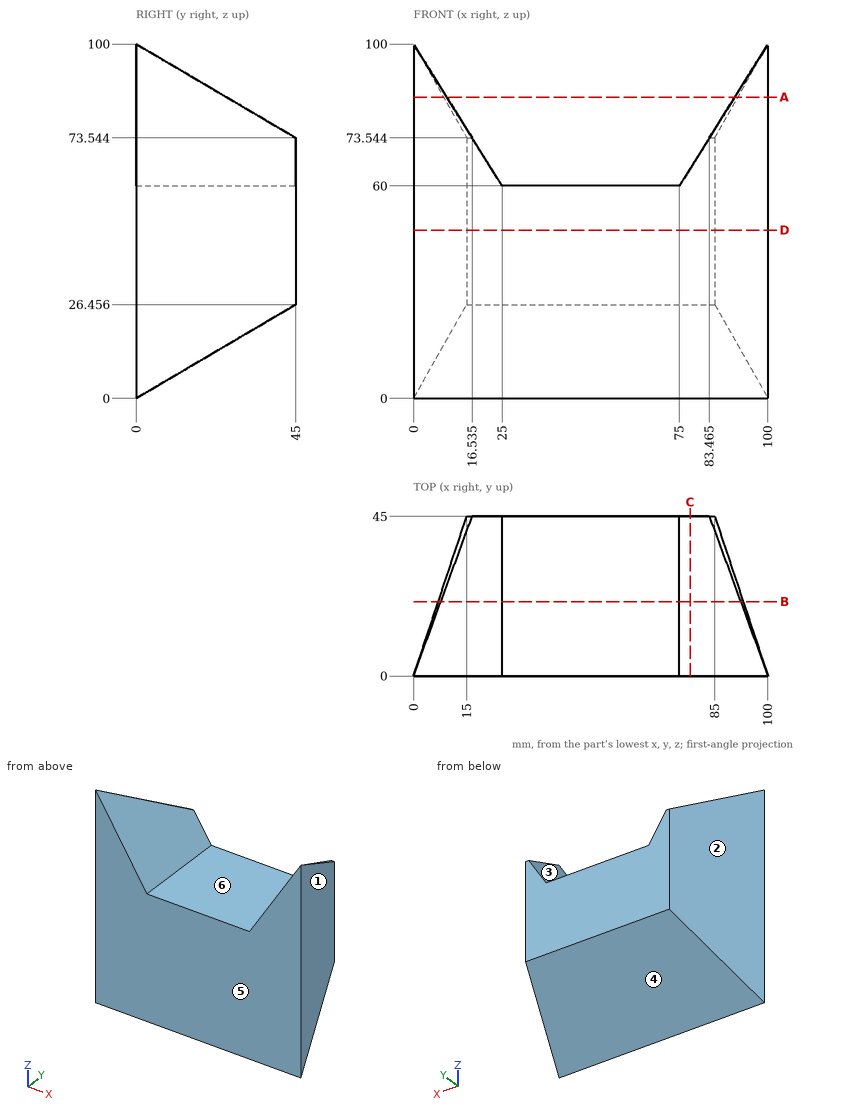
Source: three-view drawing plus pictorial views. Frame: mm from the lowest corner of the part. A direction names the side the tool comes from. Give positions to 0.01 mm unless a question says otherwise; leave off trailing zeros. Write each loop counter-clockwise with the first axis right and the second up, starting at its lowest first coordinate (ties: lowest second). Pieces come first, ordered by that corner, then holes.
(1) Mould query, pull axis X, two halves, no side actions, for the marked faces 1, 2, 3 and 4. Classes: released by +X, released by -X, zero draft, split by the parting line, or undercut.
(2) Cut plane C-C, the plane x = 78. Return loops of the section in (y, z).
(3) Access query for the marked faces 5 and 6. Directions: +Z, -Z, +X, -X, +Y, -Y. A direction counts if a zero-diameter tool reaches every point of the face in a straight line with its end or side. Return the directions, or none.
(4) Cut plane B-B, the plane y = 21. Return loops of the section in (x, z).
(5) First-contact query: P1, Ø8, axis at x = 43, y = 39, coming from the +Z side; P2, Ø1.5, axis at x = 47, y = 24, coming from the -Z side; P3, Ø6, axis at y = 24, z = 70.5, coming from the +X side. Flat tips, straight axial feed; report the tip coordinate or a pass-through.
(6) Ray query, line 1 (X direction, y = 20, z = 88); line 2 (X direction, y = 16.5, z = 70); line 3 (X direction, y = 21.5, z = 15.5). Return the intervals inside material, ascending.
(7) Cut plane A-A, the plane z = 85. Return loops of the section in (x, y) (1 decimal), then the cut area to 3 significant figures.
(8) Cut plane D-D, the plane z = 47.5. Return loops of the section in (x, y), then the cut area to 4 significant figures.
Values follow:
1. face 1: released by +X
1. face 2: released by -X
1. face 3: undercut
1. face 4: zero draft
2. outline: (0, 0) - (45, 26.46) - (45, 64.8) - (0, 64.8) - close
3. face 5: +Z, -Z, +X, -X, -Y
3. face 6: +Z, +Y, -Y
4. outline: (7, 12.35) - (93, 12.35) - (93, 87.65) - (92.28, 87.65) - (75, 60) - (25, 60) - (7.72, 87.65) - (7, 87.65) - close
5. P1: stops at z = 60
5. P2: stops at z = 13.67
5. P3: stops at x = 93
6. line 1: x = 6.67 to 7.5, 92.5 to 93.33
6. line 2: x = 5.5 to 18.75, 81.25 to 94.5
6. line 3: x = 7.17 to 92.83
7. outline: (0, 0) - (9.4, 0) - (9.4, 25.5) - (8.5, 25.5) - close; (90.6, 0) - (100, 0) - (91.5, 25.5) - (90.6, 25.5) - close
7. area: 261 mm2
8. outline: (0, 0) - (100, 0) - (85, 45) - (15, 45) - close
8. area: 3,825 mm2
